Input: part model. Units: mm. Frame: model coordinates. A direction names the side the tool comes from. Round coordinates to 2 decimals unless told otherwise and drop trailing zeros. Write each loop counter-clockwise with the first axis right and the second up, starting at its lowest first coordinate (ties: lowest second). Pieces come first, ordered by that corner, then holes. Notation, with made-up numbers: (49, 82.25) -> (61, 82.25) arc R25 ccw to (61, 103.25) -> close; hole circle Ø8 at (-32, 32). An arc over 180 degrees is marked (long way). Write item = value, one per line.
```python
from build123d import *

# Parameters (mm, degrees)
F0_W      = 1346.2
F0_H      = 787.4
F1_DEPTH  = 254
F2_T      = -25.4
F3_W      = 1270
F3_H      = 254
F4_DEPTH  = 279.4
F5_T      = -25.4
F6_W      = 25.4
F6_H      = 254
F7_DEPTH  = 228.6
F8_W      = 63.5
F8_H      = 127
F9_DEPTH  = 25.4
F10_W     = 25.4
F10_H     = 254
F11_DEPTH = 228.6
F12_W     = 63.5
F12_H     = 127
F13_DEPTH = 25.4
F14_W     = 63.5
F14_H     = 127
F15_DEPTH = 25.4
F16_W     = 63.5
F16_H     = 127
F17_DEPTH = 25.4
F18_W     = 101.6
F18_H     = 127
F19_DEPTH = 25.4
F20_W     = 260.761320591
F20_H     = 131.0430763721
F21_DEPTH = 25.4
F22_W     = 124.2034286261
F22_H     = 91.7437373161
F23_DEPTH = 25.4
F24_W     = 38.1
F24_H     = 127
F25_DEPTH = 25.4
F26_W     = 43.4030661404
F26_H     = 204.1662087968
F27_DEPTH = 38.1
F28_W     = 217.1396613121
F28_H     = 47.6633155483
F29_DEPTH = 38.1
F30_W     = 126.3566912651
F30_H     = 47.6633155483
F31_DEPTH = 38.1
F32_W     = 253.5540759563
F32_H     = 47.6633155483
F33_DEPTH = 38.1
F34_W     = 206.0110867023
F34_H     = 100.5776971579
F35_DEPTH = 38.1
F36_W     = 89.4355172336
F36_H     = 266.5195167065
F37_DEPTH = 38.1
F38_R     = 105.778257903
F39_DEPTH = 38.1
F40_R     = 157.6742046587
F41_DEPTH = 38.1


# Not quite as in the source:
# - a shell that OpenCascade refuses in one call is made with other operations: the cavity is built on its own and cut out


with BuildPart() as f1:
    # F0 (on Top) → F1 (new body)
    with BuildSketch(Plane.XY):
        with Locations((-0.1443736255, 12.1287457604)):
            Rectangle(F0_W, F0_H)
    extrude(amount=F1_DEPTH)

    # F2
    f2_openings = [f1.faces().sort_by_distance(p)[0] for p in [
        (-0.144374, 12.128746, 254),
    ]]
    offset(amount=F2_T, openings=f2_openings)

    # F3 (on face) → F4 (join)
    with BuildSketch(Plane(origin=(0, 405.8287457604, 0), x_dir=(-1, 0, 0), z_dir=(0, 1, 0))):
        with Locations((-37.9556263745, 127)):
            Rectangle(F3_W, F3_H)
    extrude(amount=F4_DEPTH)

    # F5: a shell. OpenCascade refuses it in one call, so the cavity is built on its own and cut out:
    # the body offset inwards by the wall thickness, plus a prism from it out through each open face.
    f5_core = offset(f1.part, amount=F5_T, kind=Kind.INTERSECTION, mode=Mode.PRIVATE)
    f5_exits = [f5_core.faces().sort_by_distance(p)[0] for p in [
        (37.955626, 532.828746, 228.6),
    ]]
    add(f5_core, mode=Mode.SUBTRACT)
    extrude(f5_exits, amount=-F5_T, mode=Mode.SUBTRACT)

    # F6 (on face) → F7 (join)
    with BuildSketch(Plane.XY.offset(25.4)):
        with Locations((-254.1443736255, 532.8287457604)):
            Rectangle(F6_W, F6_H)
    extrude(amount=F7_DEPTH)

    # F8 (on face) → F9 (cut)
    with BuildSketch(Plane.YZ.offset(-241.4443736255)):
        with Locations((463.9602367878, 88.9)):
            Rectangle(F8_W, F8_H)
    extrude(amount=-F9_DEPTH, mode=Mode.SUBTRACT)

    # F10 (on face) → F11 (join)
    with BuildSketch(Plane.XY.offset(25.4)):
        with Locations((76.0556263745, 532.8287457604)):
            Rectangle(F10_W, F10_H)
    extrude(amount=F11_DEPTH)

    # F12 (on face) → F13 (cut)
    with BuildSketch(Plane.XZ.offset(-380.4287457604)):
        with Locations((-102.9241020679, 88.9)):
            Rectangle(F12_W, F12_H)
    extrude(amount=-F13_DEPTH, mode=Mode.SUBTRACT)

    # F14 (on face) → F15 (cut)
    with BuildSketch(Plane.XZ.offset(-380.4287457604)):
        with Locations((146.6235657334, 88.9)):
            Rectangle(F14_W, F14_H)
        with Locations((507.9058175087, 88.9)):
            Rectangle(F14_W, F14_H)
    extrude(amount=-F15_DEPTH, mode=Mode.SUBTRACT)

    # F16 (on face) → F17 (cut)
    with BuildSketch(Plane(origin=(0, -356.1712542396, 0), x_dir=(-1, 0, 0), z_dir=(0, 1, 0))):
        with Locations((400.1246755123, 88.9)):
            Rectangle(F16_W, F16_H)
    extrude(amount=-F17_DEPTH, mode=Mode.SUBTRACT)

    # F18 (on face) → F19 (cut)
    with BuildSketch(Plane(origin=(647.5556263745, 0, 0), x_dir=(0, -1, 0), z_dir=(-1, 0, 0))):
        with Locations((-102.9611633539, 88.9)):
            Rectangle(F18_W, F18_H)
    extrude(amount=-F19_DEPTH, mode=Mode.SUBTRACT)

    # F20 (on face) → F21 (cut)
    with BuildSketch(Plane.XZ.offset(-380.4287457604)):
        with Locations((327.1993100643, 154.4215381861)):
            Rectangle(F20_W, F20_H)
    extrude(amount=-F21_DEPTH, mode=Mode.SUBTRACT)

    # F22 (on face) → F23 (cut)
    with BuildSketch(Plane(origin=(647.5556263745, 0, 0), x_dir=(0, -1, 0), z_dir=(-1, 0, 0))):
        with Locations((211.2211957574, 134.7718686581)):
            Rectangle(F22_W, F22_H)
    extrude(amount=-F23_DEPTH, mode=Mode.SUBTRACT)

    # F24 (on face) → F25 (cut)
    with BuildSketch(Plane.XZ.offset(-380.4287457604)):
        with Locations((-618.1262156487, 88.9)):
            Rectangle(F24_W, F24_H)
    extrude(amount=-F25_DEPTH, mode=Mode.SUBTRACT)

    # F26 (on face) → F27 (join)
    with BuildSketch(Plane.XY.offset(25.4)):
        Polygon((647.5556263745, 380.4287457604), (539.6558175087, 380.4287457604), (539.6558175087, 332.765430212), (604.1525602341, 332.765430212), (604.1525602341, 209.5392942429), (647.5556263745, 209.5392942429), align=None)
        with Locations((625.8540933043, -49.9219410445)):
            Rectangle(F26_W, F26_H)
        Polygon((647.5556263745, -356.1712542396), (647.5556263745, -200.4013210535), (604.1525602341, -200.4013210535), (604.1525602341, -305.9601783752), (539.6558175087, -305.9601783752), (539.6558175087, -356.1712542396), align=None)
    extrude(amount=F27_DEPTH)

    # F28 (on face) → F29 (join)
    with BuildSketch(Plane.XY.offset(25.4)):
        with Locations((336.6870582104, 356.5970879862)):
            Rectangle(F28_W, F28_H)
    extrude(amount=F29_DEPTH)

    # F30 (on face) → F31 (join)
    with BuildSketch(Plane.XY.offset(25.4)):
        with Locations((25.5772807419, 356.5970879862)):
            Rectangle(F30_W, F30_H)
    extrude(amount=F31_DEPTH)

    # F32 (on face) → F33 (join)
    with BuildSketch(Plane.XY.offset(25.4)):
        with Locations((-379.1270405054, 356.5970879862)):
            Rectangle(F32_W, F32_H)
    extrude(amount=F33_DEPTH)

    # F34 (on face) → F35 (join)
    with BuildSketch(Plane.XY.offset(25.4)):
        with Locations((-395.1756507158, -178.2315000892)):
            Rectangle(F34_W, F34_H)
    extrude(amount=F35_DEPTH)

    # F36 (on face) → F37 (join)
    with BuildSketch(Plane.XY.offset(25.4)):
        with Locations((-603.1266150087, 30.4604619741)):
            Rectangle(F36_W, F36_H)
    extrude(amount=F37_DEPTH)

    # F38 (on face) → F39 (join)
    with BuildSketch(Plane.XY.offset(25.4)):
        with Locations((-397.5111842155, 0)):
            Circle(F38_R)
    extrude(amount=F39_DEPTH)

    # F40 (on face) → F41 (join)
    with BuildSketch(Plane.XY.offset(25.4)):
        with Locations((36.9560047984, -29.6728350222)):
            Circle(F40_R)
    extrude(amount=F41_DEPTH)


solid = f1.part
```
1) Access query for faces 5 (the face through (-381, 357, 63.5)), 6 (the face through (672.956, 144, 153)), 7 (the face through (-597.044, 544, 125)). Directions: +Z, -Z, +X, -X, +Y, -Y. A direction counts if a zero-diameter tool reaches every point of the face in a straight line with its end or side. Return the directions, or none.
Solutions:
face_5 = +Z
face_6 = +Z, -Z, +X, +Y, -Y
face_7 = +Z, -Z, -X, +Y
2) Cut plane C-C (x = 417). Return the cut outline in (y, z), and give its area (3 significant figures).
Solutions:
outline = (-381.57, 0) -> (685.23, 0) -> (685.23, 254) -> (659.83, 254) -> (659.83, 25.4) -> (405.83, 25.4) -> (405.83, 88.9) -> (380.43, 88.9) -> (380.43, 63.5) -> (332.77, 63.5) -> (332.77, 25.4) -> (-356.17, 25.4) -> (-356.17, 254) -> (-381.57, 254) -> close; (380.43, 219.94) -> (405.83, 219.94) -> (405.83, 254) -> (380.43, 254) -> close
area = 43,000 mm^2
3) First-contact query: P1, Ø24, axis at x = 388, y = 366.5, coming from the +Z side; P2, Ø8, axis at x = -44.5, y = 128, coming from the +Z side; P3, Ø6, axis at y = 96.5, z = 148, coming from the +X side. Flat tips, straight axial feed; report the tip coordinate or a pass-through.
Solutions:
P1 = 63.5
P2 = 25.4
P3 = -647.84
4) Cut plane B-B (z = 203). Return the cut outline in (x, y), and give its area (3 significant figures).
Solutions:
outline = (-673.24, -381.57) -> (672.96, -381.57) -> (672.96, 685.23) -> (-597.04, 685.23) -> (-597.04, 405.83) -> (-673.24, 405.83) -> close; hole (-647.84, -356.17) -> (647.56, -356.17) -> (647.56, 380.43) -> (457.58, 380.43) -> (457.58, 405.83) -> (647.56, 405.83) -> (647.56, 659.83) -> (88.76, 659.83) -> (88.76, 405.83) -> (196.82, 405.83) -> (196.82, 380.43) -> (-647.84, 380.43) -> close; hole (-571.64, 405.83) -> (-266.84, 405.83) -> (-266.84, 659.83) -> (-571.64, 659.83) -> close; hole (-241.44, 405.83) -> (63.36, 405.83) -> (63.36, 659.83) -> (-241.44, 659.83) -> close
area = 157,000 mm^2
5) Cut plane D-D (y = 298). Return the cut outline in (x, z).
Solutions:
outline = (-673.24, 0) -> (672.96, 0) -> (672.96, 254) -> (647.56, 254) -> (647.56, 63.5) -> (604.15, 63.5) -> (604.15, 25.4) -> (-647.84, 25.4) -> (-647.84, 254) -> (-673.24, 254) -> close
6) Draft query along Y for faces 1 (the face through (9, 144, 0)), 2 (the face through (-10, -381.571, 125)), 3 (the face through (-644, 405.829, 125)), 4 (the face through (-153, 380.429, 163)). Return one class per face: +Y half, -Y half, draft (parallel to the pull), parting line (faces both ways), or undercut.
Solutions:
face_1 = draft
face_2 = -Y half
face_3 = +Y half
face_4 = undercut
7) Cut plane A-A (y = 460). Return the cut outline in (x, z).
Solutions:
outline = (-597.04, 0) -> (672.96, 0) -> (672.96, 254) -> (647.56, 254) -> (647.56, 25.4) -> (88.76, 25.4) -> (88.76, 254) -> (63.36, 254) -> (63.36, 25.4) -> (-571.64, 25.4) -> (-571.64, 254) -> (-597.04, 254) -> close; (-266.84, 152.4) -> (-241.44, 152.4) -> (-241.44, 254) -> (-266.84, 254) -> close
8) Line query: L1, parallel to Y at x = 577, z = 210.5; L2, parallel to X at y = 495, z = 157.5; L3, parallel to X at y = 465.5, z = 38.5. Output: solid intervals per line, ascending. Write a range as from..to.
Solutions:
L1 = -381.57..-356.17, 380.43..405.83, 659.83..685.23
L2 = -597.04..-571.64, -266.84..-241.44, 63.36..88.76, 647.56..672.96
L3 = -597.04..-571.64, 63.36..88.76, 647.56..672.96
